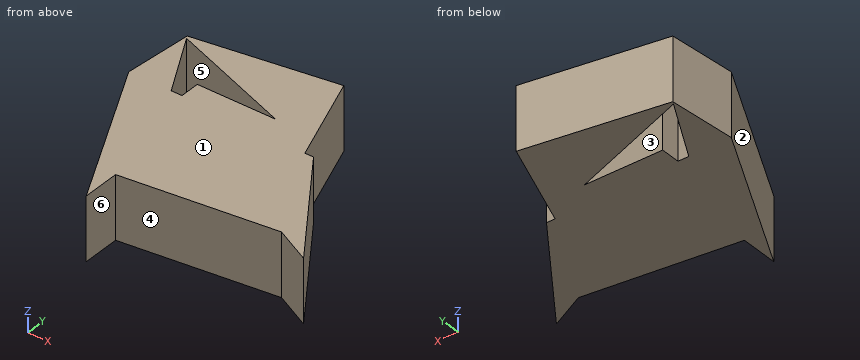
```python
from build123d import *

# Parameters (mm, degrees)
F1_DEPTH = 25


with BuildPart() as f1:
    # F0 (on Top) → F1 (new body)
    with BuildSketch(Plane.XY):
        Polygon((-40.994822979, 55.9171624482), (-43.3357991278, 29.2011853307), (-26.4946625571, 29.2011853307), (-40.3697645688, 54.765516832), align=None)
        Polygon((-26.4946625571, 29.2011853307), (-43.3357991278, 29.2011853307), (-11.9600594044, -32.6183438301), (-11.9600594044, -17.7071020007), (-15.0134380226, 8.0474792324), align=None)
        Polygon((-22.2115386277, 29.2011853307), (-26.4946625571, 29.2011853307), (-15.0134380226, 8.0474792324), (31.386833638, 17.0857999474), (27.4783183213, 27.9585812241), (8.8535510004, 27.9585812241), (8.8535510004, 36.9674563408), (-22.2115386277, 36.9674563408), align=None)
        Polygon((14.3010364845, 64.6153911948), (-40.994822979, 55.9171624482), (-40.3697645688, 54.765516832), (8.8535510004, 36.9674563408), align=None)
        Polygon((31.386833638, 17.0857999474), (-15.0134380226, 8.0474792324), (-11.9600594044, -17.7071020007), (48.3062155545, -10.56213025), align=None)
        Polygon((27.4783183213, 27.9585812241), (14.3010364845, 64.6153911948), (8.8535510004, 36.9674563408), (8.8535510004, 27.9585812241), align=None)
        Polygon((27.4783183213, 27.9585812241), (31.386833638, 17.0857999474), (48.3062155545, -10.56213025), (62.5961571932, -17.7071020007), (30.9097617865, 27.9585812241), align=None)
    extrude(amount=F1_DEPTH)


solid = f1.part
```
CAD build for the part. Positions are in the model's coordinates, mm. Face numbers are marked on the shaded views. A direction names the side the tool comes from. Coordinates: 2 decimals unless noted, no trailing zeros. Write each loop counter-clockwise with the first axis right and the second up, starting at its lowest first coordinate (ties: lowest second). Pieces come first, ordered by that corner, then holes.
(1) Flat gauge pins, fed straight in: pin 1 (1 mm diameter, centred on x = 29.5, z = 14.5, fed in from +Y); pin 2 (1.5 mm diameter, centred on y = 14, z = 4, fed in from +X); pin 3 (2.5 mm diameter, centred on y = 31.5, z = 17, fed in from -X). Where does each tip first touch, or does it go through?
(2) Two-plate mould, pull along X, no slides. Class the marked faces 1, 2 and 3: +X half, -X half, draft (parallel to the pull), parting line (faces both ways), or undercut.
(3) Cut at C-C, the plane x = -9.5. List the corners of the cut face in (y, z), and give its area (3 significant figures).
(4) Cut at D-D, the plane y = -20.5. List the corners of the cut face in (x, z), and give its area (3 significant figures).
(5) Cut at A-A, the plane z = 7.5. List the corners of the cut face in (x, y), and give its area (3 significant figures).
(6) Drill centre lines: probe 1 along Y at (x, z) = (-15, 13); probe 2 along Y at (x, z) = (-12.5, 18.5); probe 3 along X at (y, z) = (34, 8.75). Where is each one in solid material? Low to high.
(7) 3-axis set-ups, long thin cutter, end or side, ignore diameter. For the marked faces 4, 5 and 6: which of +Z, -Z, +X, -X, +Y, -Y reach the whole face in a straight line?
(8) Cut at B-B, the plane y = 44. List the corners of the cut face in (x, z), and give its area (3 significant figures).
Geometry says:
1. pin 1: stops at y = 27.96
1. pin 2: stops at x = 41.12
1. pin 3: stops at x = -43.24
2. face 1: draft
2. face 2: -X half
2. face 3: undercut
3. outline: (-17.42, 0) - (36.97, 0) - (36.97, 25) - (-17.42, 25) - close; (43.6, 0) - (60.87, 0) - (60.87, 25) - (43.6, 25) - close
3. area: 1,790 mm2
4. outline: (-18.11, 0) - (-11.96, 0) - (-11.96, 25) - (-18.11, 25) - close
4. area: 154 mm2
5. outline: (-43.34, 29.2) - (-11.96, -32.62) - (-11.96, -17.71) - (48.31, -10.56) - (62.6, -17.71) - (30.91, 27.96) - (27.48, 27.96) - (14.3, 64.62) - (-40.99, 55.92) - close; hole (-40.37, 54.77) - (-26.49, 29.2) - (-22.21, 29.2) - (-22.21, 36.97) - (8.85, 36.97) - close
5. area: 5,010 mm2
6. probe 1: y = -26.63 to 36.97, 45.59 to 60.01
6. probe 2: y = -31.55 to 36.97, 44.69 to 60.4
6. probe 3: x = -42.92 to -29.1, -22.21 to 25.31
7. face 4: +Z, -Z, -Y
7. face 5: +Z, -Z
7. face 6: +Z, -Z, +X, -Y
8. outline: (-42.04, 0) - (-34.53, 0) - (-34.53, 25) - (-42.04, 25) - close; (-10.6, 0) - (21.71, 0) - (21.71, 25) - (-10.6, 25) - close
8. area: 996 mm2
